```python
from build123d import *

# Parameters (mm, degrees)
ESBO_O1_R                = 20.4
ESBO_O1_R_2              = 4.25
RESSALTO_EXTRUS_O1_DEPTH = 10
CORTE_EXTRUS_O1_DEPTH    = 4.5
ESBO_O5_R                = 15
ESBO_O5_R_2              = 4.25
RESSALTO_EXTRUS_O2_DEPTH = 13


with BuildPart() as part:
    # Esboço1 → Ressalto-extrusão1 (new body)
    with BuildSketch(Plane.XY):
        Circle(ESBO_O1_R)
        Circle(ESBO_O1_R_2, mode=Mode.SUBTRACT)
    extrude(amount=RESSALTO_EXTRUS_O1_DEPTH)

    # Esboço2 → Corte-extrusão1 (cut)
    with BuildSketch(Plane.XY.offset(10)):
        Polygon((3.810511777, -6.6), (7.621023553, 0), (3.810511777, 6.6), (-3.810511777, 6.6), (-7.621023553, 0), (-3.810511777, -6.6), align=None)
    extrude(amount=-CORTE_EXTRUS_O1_DEPTH, mode=Mode.SUBTRACT)

    # Esboço5 → Ressalto-extrusão2 (add)
    with BuildSketch(Plane(origin=(0, 0, 0), x_dir=(-1, 0, 0), z_dir=(0, 0, -1))):
        Circle(ESBO_O5_R)
        Circle(ESBO_O5_R_2, mode=Mode.SUBTRACT)
    extrude(amount=RESSALTO_EXTRUS_O2_DEPTH)


solid = part.part
```
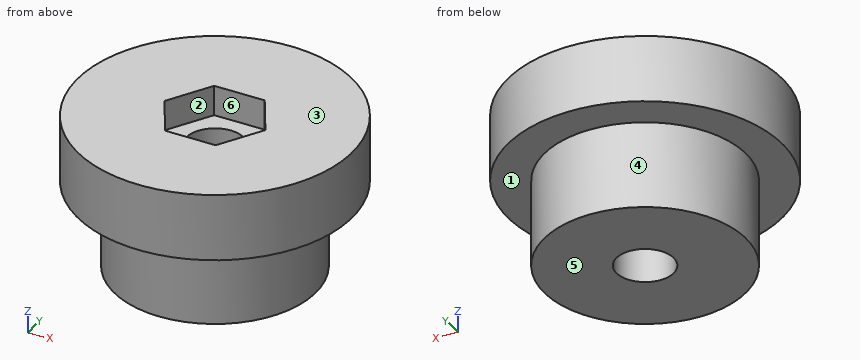
The listing builds one solid part. Answer for the finished solid, in the listing's coordinates (mm). Face numbers are marked on the shaded views. A direction names the side the tool comes from. Coordinates: 2 decimals unless noted, no trailing zeros. Loops run counter-clockwise (first coordinate to the right, second up) from the corner with the lowest first, then second, coordinate; pieces in that order, holes last. Notation, with made-up numbers: (52.5, 27) -> (58.5, 27) arc R23 cw to (58.5, 43) -> close; hole circle Ø3 at (-1, 34.25). An arc over 180 degrees is marked (long way). Return JSON: item names as keys, results as strings. Group by question number.
(1) A cutting plane is placed at D-D on x = -10. Write down the section's boundary in (y, z).
(2) A cutting plane is placed at A-A on x = 0. Write down the section's boundary in (y, z).
(3) Determine the mould class of the marked faces 4, 5 and 6 for opening direction X: released by +X, released by -X, zero draft, split by the parting line, or undercut.
(4) Given pin 1 Ø4 at (x, y) = (3.5, -2) entering from +Z; pin 2 Ø10 at (x, z) = (-1.5, -3) entering from -Y; pin 3 Ø1.3 at (x, z) = (-1, 8.5) entering from +Y, each flat-ended and moving along its own axis, determine where each tip first touches the part or whether it passes through.
(5) A cutting plane is placed at C-C on y = -1. Write down the section's boundary in (x, z), and give its area (3 significant figures).
(6) A cutting plane is placed at B-B on z = 7.75. Write down the section's boundary in (x, y), and give its area (3 significant figures).
(7) Which of the six approach directions +Z, -Z, +X, -X, +Y, -Y give full straight-line access (tool end or side, diameter ignored) to the marked faces 1, 2 and 3?
(8) Find the intervals of material crossed by probe 1 along Y at (x, z) = (0, -3.5); probe 2 along Y at (x, z) = (0, 1.75); probe 3 along Z at (x, y) = (13, 10), in increasing order. Write a range as from..to.
The answers:
{
 "1": {"outline": "(-17.78, 0) -> (-11.18, 0) -> (-11.18, -13) -> (11.18, -13) -> (11.18, 0) -> (17.78, 0) -> (17.78, 10) -> (-17.78, 10) -> close"},
 "2": {"outline": "(-20.4, 0) -> (-15, 0) -> (-15, -13) -> (-4.25, -13) -> (-4.25, 5.5) -> (-6.6, 5.5) -> (-6.6, 10) -> (-20.4, 10) -> close; (4.25, -13) -> (15, -13) -> (15, 0) -> (20.4, 0) -> (20.4, 10) -> (6.6, 10) -> (6.6, 5.5) -> (4.25, 5.5) -> close"},
 "3": {"face 4": "split by the parting line", "face 5": "zero draft", "face 6": "undercut"},
 "4": {"pin 1": "stops at z = 5.5", "pin 2": "stops at y = -20.4", "pin 3": "stops at y = 20.4"},
 "5": {"outline": "(-20.38, 0) -> (-14.97, 0) -> (-14.97, -13) -> (-4.13, -13) -> (-4.13, 5.5) -> (-7.04, 5.5) -> (-7.04, 10) -> (-20.38, 10) -> close; (4.13, -13) -> (14.97, -13) -> (14.97, 0) -> (20.38, 0) -> (20.38, 10) -> (7.04, 10) -> (7.04, 5.5) -> (4.13, 5.5) -> close", "area": "580 mm^2"},
 "6": {"outline": "circle Ø40.8 at (0, 0); hole (-7.62, 0) -> (-3.81, -6.6) -> (3.81, -6.6) -> (7.62, 0) -> (3.81, 6.6) -> (-3.81, 6.6) -> close", "area": "1,160 mm^2"},
 "7": {"face 1": "-Z", "face 2": "+Z", "face 3": "+Z, +X, -X, +Y, -Y"},
 "8": {"probe 1": "y = -15..-4.25, 4.25..15", "probe 2": "y = -20.4..-4.25, 4.25..20.4", "probe 3": "z = 0..10"}
}
